Geometry: final body of the model. Coordinates: model frame, mm. A direction names the side the tool comes from. Give positions to 0.01 mm unless a question says otherwise; leave off trailing zeros. Loops run counter-clockwise (first coordinate to the right, second up) from the corner with the lowest first, then second, coordinate; pieces in that order, holes last. Notation, with made-up numbers: (49.25, 51) - (56.25, 51) arc R19 ccw to (56.25, 74) - close; hole circle Ø9 at (83, 24). An arc over 180 degrees is marked (long way). Use CSV: the item, a comma, the result in double quotes. Start each with the question number.
```python
from build123d import *

# Parameters (mm, degrees)
F1_R     = 3.5
F2_DEPTH = 15
F3_R     = 0.5
F4_DEPTH = 5
F0_R     = 3.5
F5_DEPTH = 25.4
F6_R     = 0.5
F7_DEPTH = 5


with BuildPart() as f2:
    # F1 (on face) → F2 (new body)
    with BuildSketch(Plane.XZ):
        Circle(F1_R)
    extrude(amount=F2_DEPTH)

    # F3 (on face) → F4 (join)
    with BuildSketch(Plane.XZ):
        Circle(F3_R)
    extrude(amount=F4_DEPTH)

    # F0 (on Front) → F5 (join)
    with BuildSketch(Plane.XZ):
        Circle(F0_R)
    extrude(amount=F5_DEPTH)

    # F6 (on face) → F7 (join)
    with BuildSketch(Plane(origin=(0, 0, 0), x_dir=(-1, 0, 0), z_dir=(0, 1, 0))):
        Circle(F6_R)
    extrude(amount=F7_DEPTH)


solid = f2.part
```
Item 1: Section A-A (z = 0). Output: boundary loops of the cut face in (x, y), plus the area to 3 significant figures.
Item 2: Section C-C (y = 0.5). Output: boundary loops of the cut face in (x, z), plus the area to 3 significant figures.
Item 3: Section D-D (z = -1.25). Output: boundary loops of the cut face in (x, y).
Item 4: Ray query, probe 1 along Y at (x, z) = (-2, -2); probe 2 along X at (y, z) = (-4, 3); probe 3 along X at (y, z) = (-6, 2.5). Return the intervals inside material, ascending.
Item 5: Reachability of faces 1 (the flat face through (0, 5, 0)), 2 (the cylindrical face through (0.108, 2.465, -0.488)) from +Z, -Z, +X, -X, +Y, -Y: full face, straight path, thin tool, end or side. Return the list, or none.
Item 6: Section B-B (x = 0). Output: boundary loops of the cut face in (y, z).
Item 7: Pin query (flat end, axial travel): pin 1 Ø2 at (x, z) = (-1, 1.5) entering from +Y; pin 2 Ø1.5 at (x, y) = (-1.5, -17) entering from +Z. Return the tip coordinate at first contact, or that it passes through.
Outcome:
1,outline,"(-3.5, -25.4) - (3.5, -25.4) - (3.5, 0) - (0.5, 0) - (0.5, 5) - (-0.5, 5) - (-0.5, 0) - (-3.5, 0) - close"
1,area,"183 mm2"
2,outline,"circle Ø1 at (0, 0)"
2,area,"0.785 mm2"
3,outline,"(-3.27, -25.4) - (3.27, -25.4) - (3.27, 0) - (-3.27, 0) - close"
4,probe 1,"y = -25.4 to 0"
4,probe 2,"x = -1.8 to 1.8"
4,probe 3,"x = -2.45 to 2.45"
5,face 1,"+Z, -Z, +X, -X, +Y"
5,face 2,"+Y"
6,outline,"(-25.4, -3.5) - (0, -3.5) - (0, -0.5) - (5, -0.5) - (5, 0.5) - (0, 0.5) - (0, 3.5) - (-25.4, 3.5) - close"
7,pin 1,"stops at y = 0"
7,pin 2,"stops at z = 3.42"
